Design review of the part built by this model. Coordinates are the model's own, in mm. A direction names the side the tool comes from. Give positions to 0.01 mm unless a question says otherwise; leave off trailing zeros. Loops run counter-clockwise (first coordinate to the right, second up) from the corner with the lowest first, then second, coordinate; pieces in that order, holes last. Notation, with made-up numbers: (60, 74) -> (87, 74) arc R10 ccw to (87, 92) -> close; hole circle Ø8 at (-33.75, -40). An arc over 180 degrees is marked (long way). Use CSV: the item, a comma, the result in double quotes. Start each with the question number.
Item 1: The part is to be moulded in two halves that separate along X. For faces 1 (the face through (107.95, 5, 0)), 2 (the face through (102, 2, 19.05)), 3 (the face through (-104.14, 8, 0)), say which applies: +X half, -X half, draft (parallel to the pull), parting line (faces both ways), or undercut.
Item 2: We need section D-D (x = 56.5). State the section outline as (y, z) points, plus the area to 3 significant figures.
Item 3: Wall thickness on line 1 along X through (y, z) = (5, -8); line 2 along X through (y, z) = (3, 14); line 3 along Z through (x, y) = (-76.5, 3): over which ranges is each line inside the solid? List them lowest first. Write a range as from..to.
Item 4: We need section B-B (y = 9.25). State the section outline as (x, z) points.
Item 5: We need section A-A (z = -14.5). State the section outline as (x, y) points (3 decimals).
Item 6: We need section C-C (z = 1). State the section outline as (x, y) points.
Item 7: For faces 4 (the face through (95.25, 2, -15)), 5 (the face through (-95.25, 2, 15)), 6 (the face through (-1, 3.81, 0)), list the 3-axis set-ups (+Z, -Z, +X, -X, +Y, -Y) from which the entire face can be reached by the end or side of a thin tool; tool diameter is ignored.
Item 8: Clearance check with flat-ended pins moving along their axes: pin 1 (1.1 mm diameter, centred on x = -22, y = 1.5, fed in from -Z); pin 2 (1.9 mm diameter, centred on x = 2.5, y = 1.5, fed in from +Z); pin 3 (1.5 mm diameter, centred on x = -38, z = -6.5, fed in from +Y). State where each tip first meets the part, or that it passes through.
from build123d import *

# Parameters (mm, degrees)
BOSS_EXTRUDE1_DEPTH = 3.81
BOSS_EXTRUDE2_DEPTH = 3.81
FILLET1_R           = 1.27
FILLET2_R           = 1.27


with BuildPart() as part:
    # Sketch1 → Boss-Extrude1 (new body)
    with BuildSketch(Plane(origin=(0, 0, 0), x_dir=(1, 0, 0), z_dir=(0, 1, 0))):
        Polygon((95.25, 10.16), (-95.25, 10.16), (-95.25, 19.05), (-107.95, 19.05), (-107.95, -19.05), (-95.25, -19.05), (-95.25, -10.16), (95.25, -10.16), (95.25, -19.05), (107.95, -19.05), (107.95, 19.05), (95.25, 19.05), align=None)
    extrude(amount=BOSS_EXTRUDE1_DEPTH)

    # Sketch2 → Boss-Extrude2 (add)
    with BuildSketch(Plane.ZY.offset(107.95)):
        Polygon((-19.05, 0), (-19.05, 3.81), (-6.35, 12.7), (6.35, 12.7), (19.05, 3.81), (19.05, 0), align=None)
    boss_extrude2 = extrude(amount=-BOSS_EXTRUDE2_DEPTH)

    # Mirror1: Boss-Extrude2 across plane
    add(boss_extrude2.mirror(Plane(origin=(0, 0, 0), x_dir=(0, 0, 1), z_dir=(1, 0, 0))))

    # Fillet1
    fillet1_edges = [part.edges().sort_by_distance(p)[0] for p in [
        (-104.14, 3.81, 0),
        (-106.045, 12.7, -6.35),
        (-106.045, 12.7, 6.35),
        (104.14, 3.81, 0),
        (106.045, 12.7, 6.35),
        (106.045, 12.7, -6.35),
    ]]
    fillet(fillet1_edges, radius=FILLET1_R)

    # Fillet2
    fillet2_edges = [part.edges().sort_by_distance(p)[0] for p in [
        (-95.25, 1.905, -10.16),
        (95.25, 1.905, -10.16),
        (95.25, 1.905, 10.16),
        (-95.25, 1.905, 10.16),
    ]]
    fillet(fillet2_edges, radius=FILLET2_R)


solid = part.part
Results found:
1,face 1,"+X half"
1,face 2,"draft"
1,face 3,"undercut"
2,outline,"(0, -10.16) -> (3.81, -10.16) -> (3.81, 10.16) -> (0, 10.16) -> close"
2,area,"77.4 mm²"
3,line 1,"-107.95..-104.14, 104.14..107.95"
3,line 2,"-107.95..-95.25, 95.25..107.95"
3,line 3,"-10.16..10.16"
4,outline,"(-107.95, -11.28) -> (-104.14, -11.28) -> (-104.14, 11.28) -> (-107.95, 11.28) -> close; (104.14, -11.28) -> (107.95, -11.28) -> (107.95, 11.28) -> (104.14, 11.28) -> close"
5,outline,"(-107.95, 0) -> (-95.25, 0) -> (-95.25, 3.81) -> (-102.87, 3.81) arc R1.27 cw to (-104.14, 5.08) -> (-104.14, 6.995) -> (-107.95, 6.995) -> close; (95.25, 0) -> (107.95, 0) -> (107.95, 6.995) -> (104.14, 6.995) -> (104.14, 5.08) arc R1.27 cw to (102.87, 3.81) -> (95.25, 3.81) -> close"
6,outline,"(-107.95, 0) -> (107.95, 0) -> (107.95, 12.7) -> (104.14, 12.7) -> (104.14, 5.08) arc R1.27 cw to (102.87, 3.81) -> (-102.87, 3.81) arc R1.27 cw to (-104.14, 5.08) -> (-104.14, 12.7) -> (-107.95, 12.7) -> close"
7,face 4,"-Z, +Y, -Y"
7,face 5,"+Z, +Y, -Y"
7,face 6,"+Z, -Z, +Y"
8,pin 1,"z = -10.16"
8,pin 2,"z = 10.16"
8,pin 3,"y = 3.81"
